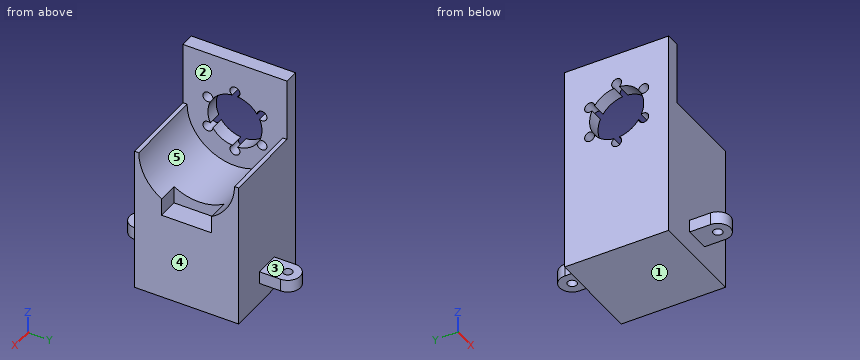
```python
from build123d import *

# Parameters (mm, degrees)
SKETCH_1_W          = 23
SKETCH_1_H          = 25
EXTRUDE_1_DEPTH     = 35
SKETCH_2_W          = 19.6
SKETCH_2_H          = 11.5
SKETCH_4_W          = 3.4
SKETCH_4_H          = 25
EXTRUDE_2_DEPTH     = 15
SKETCH_6_R          = 1.2
SKETCH_6_R_2        = 6.5
CUT_EXTRUDE_1_DEPTH = 4
SKETCH_7_W          = 5
SKETCH_7_H          = 12
CUT_EXTRUDE_3_DEPTH = 5
SKETCH_8_R          = 1.1
EXTRUDE_3_DEPTH     = 8
SKETCH_8_2_R        = 1.1
CUT_EXTRUDE_4_DEPTH = 5


with BuildPart() as part:
    # Sketch 1 → Extrude 1 (new body)
    with BuildSketch(Plane.XY):
        Rectangle(SKETCH_1_W, SKETCH_1_H)
    extrude(amount=-EXTRUDE_1_DEPTH)

    # Sketch 2 → Cut-Revolve 2 (revolve, cut)
    with BuildSketch(Plane.XY):
        with Locations((1.7, -5.75)):
            Rectangle(SKETCH_2_W, SKETCH_2_H)
    revolve(axis=Axis((11.5, 0, 0), (-1, 0, 0)), mode=Mode.SUBTRACT)

    # Sketch 4 → Extrude 2 (add)
    with BuildSketch(Plane.XY):
        with Locations((-9.8, 0)):
            Rectangle(SKETCH_4_W, SKETCH_4_H)
    extrude(amount=EXTRUDE_2_DEPTH)

    # Sketch 6 → Cut-Extrude 1 (cut)
    with BuildSketch(Plane(origin=(-8.1, 0, 0), x_dir=(0, 0, -1), z_dir=(1, 0, 0))):
        with Locations((7.5, 0)):
            Circle(SKETCH_6_R)
        with Locations((3.75, -6.495190528)):
            Circle(SKETCH_6_R)
        with Locations((-3.75, -6.495190528)):
            Circle(SKETCH_6_R)
        Circle(SKETCH_6_R_2)
        with Locations((-7.5, 0)):
            Circle(SKETCH_6_R)
        with Locations((-3.75, 6.495190528)):
            Circle(SKETCH_6_R)
        with Locations((3.75, 6.495190528)):
            Circle(SKETCH_6_R)
    extrude(amount=-CUT_EXTRUDE_1_DEPTH, mode=Mode.SUBTRACT)

    # Sketch 7 → Cut-Extrude 3 (cut)
    with BuildSketch(Plane(origin=(11.5, 0, 0), x_dir=(0, 0, -1), z_dir=(1, 0, 0))):
        with Locations((11.5, 0)):
            Rectangle(SKETCH_7_W, SKETCH_7_H)
    extrude(amount=-CUT_EXTRUDE_3_DEPTH, mode=Mode.SUBTRACT)

    # Sketch 8 → Extrude 3 (add)
    # profile 1 of 2: a face of its own
    with BuildSketch(Plane(origin=(0, 0, -35), x_dir=(-1, 0, 0), z_dir=(0, 0, -1))):
        with BuildLine():
            Line((3, 17.5), (3, 12.5))
            Line((3, 12.5), (-3, 12.5))
            Line((-3, 12.5), (-3, 17.5))
            ThreePointArc((-3, 17.5), (0, 20.5), (3, 17.5))
        make_face()
        with Locations(Location((0, 17.5, 0), (0, 0, 180))):
            Circle(SKETCH_8_R, mode=Mode.SUBTRACT)
    # profile 2 of 2: a face of its own
    with BuildSketch(Plane(origin=(0, 0, -35), x_dir=(-1, 0, 0), z_dir=(0, 0, -1))):
        with BuildLine():
            Line((-3, -17.5), (-3, -12.5))
            Line((-3, -12.5), (3, -12.5))
            Line((3, -12.5), (3, -17.5))
            ThreePointArc((3, -17.5), (0, -20.5), (-3, -17.5))
        make_face()
        with Locations((0, -17.5)):
            Circle(SKETCH_8_R, mode=Mode.SUBTRACT)
    extrude(amount=-EXTRUDE_3_DEPTH)

    # Sketch 8_2 → Cut-Extrude 4 (cut)
    # profile 1 of 2: a face of its own
    with BuildSketch(Plane(origin=(0, 0, -35), x_dir=(-1, 0, 0), z_dir=(0, 0, -1))):
        with BuildLine():
            Line((3, 17.5), (3, 12.5))
            Line((3, 12.5), (-3, 12.5))
            Line((-3, 12.5), (-3, 17.5))
            ThreePointArc((-3, 17.5), (0, 20.5), (3, 17.5))
        make_face()
        with Locations(Location((0, 17.5, 0), (0, 0, 180))):
            Circle(SKETCH_8_2_R, mode=Mode.SUBTRACT)
    # profile 2 of 2: a face of its own
    with BuildSketch(Plane(origin=(0, 0, -35), x_dir=(-1, 0, 0), z_dir=(0, 0, -1))):
        with BuildLine():
            Line((-3, -17.5), (-3, -12.5))
            Line((-3, -12.5), (3, -12.5))
            Line((3, -12.5), (3, -17.5))
            ThreePointArc((3, -17.5), (0, -20.5), (-3, -17.5))
        make_face()
        with Locations((0, -17.5)):
            Circle(SKETCH_8_2_R, mode=Mode.SUBTRACT)
    extrude(amount=-CUT_EXTRUDE_4_DEPTH, mode=Mode.SUBTRACT)


solid = part.part
```
Could you check a few things on this model? Use its own coordinates, in mm. Face numbers are marked on the shaded views. A direction names the side the tool comes from. Round coordinates to 2 decimals unless told otherwise and drop trailing zeros. Loops run counter-clockwise (first coordinate to the right, second up) from the corner with the lowest first, then second, coordinate; pieces in that order, holes last. Notation, with made-up numbers: (54.5, 20.5) -> (60.5, 20.5) arc R10 cw to (60.5, 34.5) -> close; hole circle Ø2 at (1, 23.25). An arc over 180 degrees is marked (long way). One line per question, with ' | ' between items.
(1) If I drill on probe 1 along Y at (x, z) = (-9.05, -7.5); probe 2 along Y at (x, z) = (0, -28.8); probe 3 along Y at (x, z) = (10.25, -17), over which ranges is the centre line in solid material (lowest first)?
Model answer:
probe 1: y = -12.5 to -1.2, 1.2 to 12.5 | probe 2: y = -20.5 to -18.6, -16.4 to 16.4, 18.6 to 20.5 | probe 3: y = -12.5 to 12.5
(2) For the marked faces 3, 4 and 5, which set-ups out of +Z, -Z, +X, -X, +Y, -Y let a thin tool reach every point of the face, with its end or its side?
Model answer:
face 3: +Z, +X, -X, +Y | face 4: +Z, -Z, +X, +Y, -Y | face 5: +Z, +X
(3) For pin 1 Ø6 at (x, z) = (7, -8) entering from +Y; pin 2 Ø3.5 at (x, z) = (9.5, -12.5) entering from -Y; pin 3 Ø6.5 at (x, y) = (0.5, 15) entering from +Z; pin 4 Ø5 at (y, z) = (-3, 0.5) entering from -X, each with a flat end and sliding along its axis, tell me the tip position at first contact or that it passes through.
Model answer:
pin 1: stops at y = 12.5 | pin 2: stops at y = -12.5 | pin 3: stops at z = 0 | pin 4: passes through
(4) Thinking about a two-plate mould opening in Y: for the marked faces 1 and 2, which applies, released by +Y, released by -Y, zero draft, split by the parting line, or undercut?
Model answer:
face 1: zero draft | face 2: undercut
(5) If we section it at D-D on x = 4.5: List the corners of the cut face in (y, z) for me, and give its area (3 significant figures).
Model answer:
outline: (-12.5, -35) -> (12.5, -35) -> (12.5, 0) -> (11.5, 0) arc R11.5 cw to (-11.5, 0) -> (-12.5, 0) -> close | area: 667 mm^2
(6) If we section it at B-B on z = 7.5: List the corners of the cut face in (x, y) for me, and give its area (3 significant figures).
Model answer:
outline: (-11.5, -12.5) -> (-8.1, -12.5) -> (-8.1, -1.2) -> (-11.5, -1.2) -> close; (-11.5, 1.2) -> (-8.1, 1.2) -> (-8.1, 12.5) -> (-11.5, 12.5) -> close | area: 76.8 mm^2
(7) If we section it at C-C on y = 0: List the corners of the cut face in (x, z) for me, and give its area (3 significant figures).
Model answer:
outline: (-11.5, -35) -> (11.5, -35) -> (11.5, -14) -> (6.5, -14) -> (6.5, -11.5) -> (-8.1, -11.5) -> (-8.1, -8.7) -> (-11.5, -8.7) -> close; (-11.5, 8.7) -> (-8.1, 8.7) -> (-8.1, 15) -> (-11.5, 15) -> close | area: 559 mm^2
(8) If we section it at A-A on x = 0: List the corners of the cut face in (y, z) for me, and give its area (3 significant figures).
Model answer:
outline: (-20.5, -30) -> (-18.6, -30) -> (-18.6, -27) -> (-20.5, -27) -> close; (-16.4, -30) -> (-12.5, -30) -> (-12.5, -35) -> (12.5, -35) -> (12.5, -30) -> (16.4, -30) -> (16.4, -27) -> (12.5, -27) -> (12.5, 0) -> (11.5, 0) arc R11.5 cw to (-11.5, 0) -> (-12.5, 0) -> (-12.5, -27) -> (-16.4, -27) -> close; (18.6, -30) -> (20.5, -30) -> (20.5, -27) -> (18.6, -27) -> close | area: 702 mm^2
